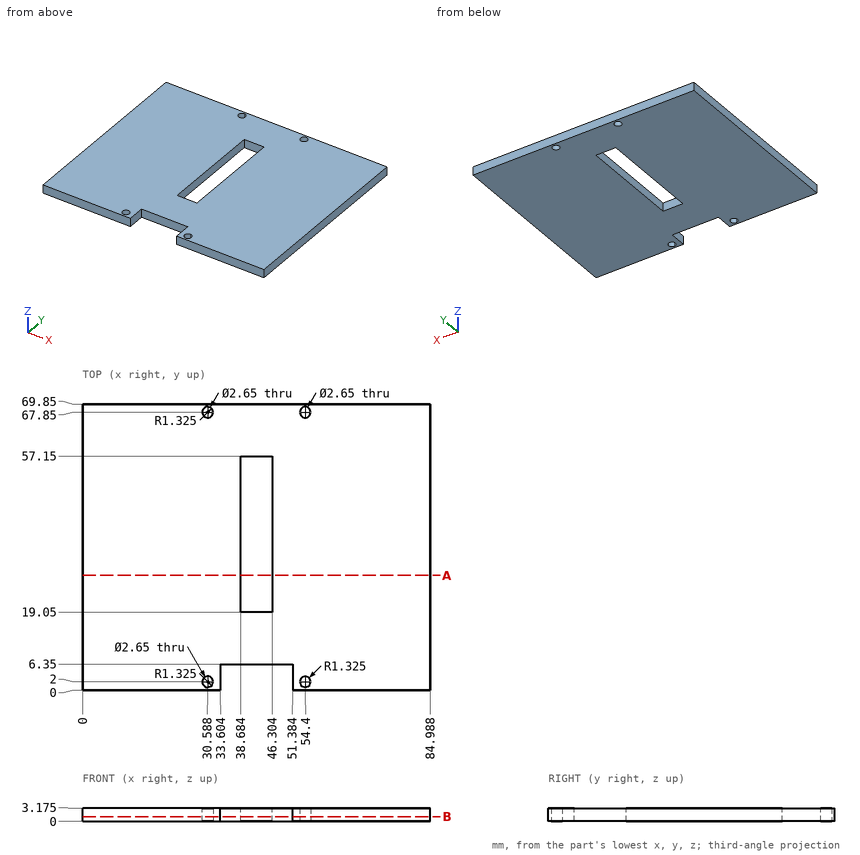
Job drawing, mm, ordinate dimensions from the low corner. One solid piece. Coordinates: 2 decimals unless noted, no trailing zeros. Write each loop counter-clockwise with the first axis right and the second up, starting at its lowest first coordinate (ties: lowest second). Pieces come first, ordered by that corner, then holes. Notation, with made-up numbers: M 8,-17.75 L 23,-17.75 A7 ccw 23,-5.75 Z; hole C 37.25,81.25 d11. An arc over 180 degrees is marked long. Answer as a JSON object with one key per item and string values. Group by question number.
1) Saw through at B-B (z = 1.05). Give the number of separate pieces and of enclosed holes in the cut face, plus the area to 3 significant figures.
2) Wall check: line 1 (X direction, y = 2, z = 2.1) (1 decimal); line 2 (X direction, y = 67.85, z = 2.35) (1 decimal); line 3 (Y direction, x = 43.5, z = 0.35). Give the ranges that are in metal, low to high. Write a range as from..to.
3) Pin check, flat tips, straight feed: pin 1 Ø1 at (x, z) = (43, 1.5) entering from -Y; pin 2 Ø1.6 at (x, y) = (30.59, 2) entering from -Z (3 decimals). Stop position of each tip, or through.
4) Saw through at A-A (y = 28). Write the cut outline in (x, z) (1 decimal).
Values follow:
{
 "1": {"separate pieces": "1", "enclosed holes": "5", "area": "5,510 mm2"},
 "2": {"line 1": "x = 0..29.3, 31.9..33.6, 51.4..53.1, 55.7..85", "line 2": "x = 0..29.3, 31.9..53.1, 55.7..85", "line 3": "y = 6.35..19.05, 57.15..69.85"},
 "3": {"pin 1": "stops at y = 6.35", "pin 2": "passes through"},
 "4": {"outline": "M 0,0 L 38.7,0 L 38.7,3.2 L 0,3.2 Z; M 46.3,0 L 85,0 L 85,3.2 L 46.3,3.2 Z"}
}
